Could you check a few things on this model? Use its own coordinates, in mm. Face numbers are marked on the shaded views. Coordinates: 2 decimals unless noted, no trailing zeros. Order: outer loops, then holes, each group sorted by start corner. A loop starts at its lowest first (then second) coordinate and runs counter-clockwise, first axis right, second up. Notation, with made-up numbers: (74.5, 69.5) -> (97.5, 69.5) arc R27 ccw to (97.5, 104.5) -> close; hole circle Ø4 at (-21.5, 67.25). An arc over 180 degrees is marked (long way). Put each result on its own line as item: value. Start each with the question number.
Q1. If we section it at D-D (z = -10.5): Please give me the cut outline in (x, y), and give its area (3 significant figures).
Q2. Please list where these lines run through material, in increasing order: line 1 along Z through (x, y) = (-6, 6.4); line 2 along X through (y, z) = (5.6, -10.5); line 3 along Z through (x, y) = (-10.5, 3.5).
Q3. We'd pull the mould along Z, two halves only. Please class the marked faces 1, 2 and 3: +Z half, -Z half, draft (parallel to the pull), parting line (faces both ways), or undercut.
Q4. If we section it at B-B (y = 3.25): Please give me the cut outline in (x, z), and give its area (3 significant figures).
Q5. If we section it at C-C (x = -12): Please give me the cut outline in (y, z), and give its area (3 significant figures).
Q6. If we section it at A-A (y = 8.5): Please give me the cut outline in (x, z).
Q7. Will these pins go through, and if not, where does the flat tip stop? pin 1 (2 mm diameter, centred on y = 1.5, z = -6.5, fed in from -X); pin 2 (0.9 mm diameter, centred on x = 5.5, z = -10, fed in from +Y).
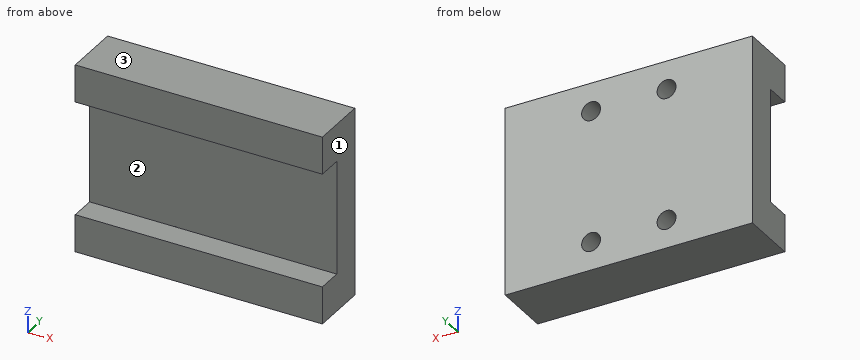
from build123d import *

# Parameters (mm, degrees)
SKETCH_1_W          = 39.3
SKETCH_1_H          = 30
EXTRUDE_1_DEPTH     = 9
SKETCH_2_W          = 39.3
SKETCH_2_H          = 18.1
CUT_EXTRUDE_1_DEPTH = 4
SKETCH_3_R          = 1.5
CUT_EXTRUDE_2_DEPTH = 5


with BuildPart() as part:
    # 草图1 → 凸台-拉伸1 (new body)
    with BuildSketch(Plane(origin=(0, 0, 0), x_dir=(1, 0, 0), z_dir=(0, 1, 0))):
        Rectangle(SKETCH_1_W, SKETCH_1_H)
    extrude(amount=EXTRUDE_1_DEPTH)

    # 草图2 → 切除-拉伸1 (cut)
    with BuildSketch(Plane.XZ):
        Rectangle(SKETCH_2_W, SKETCH_2_H)
    extrude(amount=-CUT_EXTRUDE_1_DEPTH, mode=Mode.SUBTRACT)

    # 草图3 → 切除-拉伸2 (cut)
    with BuildSketch(Plane(origin=(0, 9, 0), x_dir=(1, 0, 0), z_dir=(0, 1, 0))):
        with Locations((-6, 10.5)):
            Circle(SKETCH_3_R)
        with Locations((6, 10.5)):
            Circle(SKETCH_3_R)
        with Locations((6, -10.5)):
            Circle(SKETCH_3_R)
        with Locations((-6, -10.5)):
            Circle(SKETCH_3_R)
    extrude(amount=-CUT_EXTRUDE_2_DEPTH, mode=Mode.SUBTRACT)


solid = part.part
The answers:
1. outline: (-19.65, 0) -> (19.65, 0) -> (19.65, 9) -> (7.5, 9) -> (7.5, 4) -> (4.5, 4) -> (4.5, 9) -> (-4.5, 9) -> (-4.5, 4) -> (-7.5, 4) -> (-7.5, 9) -> (-19.65, 9) -> close
1. area: 324 mm^2
2. line 1: -15 to -12, -9 to 9, 12 to 15
2. line 2: -19.65 to -7.5, -4.5 to 4.5, 7.5 to 19.65
2. line 3: -15 to -9.05, 9.05 to 15
3. face 1: draft
3. face 2: undercut
3. face 3: +Z half
4. outline: (-19.65, -15) -> (19.65, -15) -> (19.65, -9.05) -> (-19.65, -9.05) -> close; (-19.65, 9.05) -> (19.65, 9.05) -> (19.65, 15) -> (-19.65, 15) -> close
4. area: 468 mm^2
5. outline: (0, -15) -> (9, -15) -> (9, 15) -> (0, 15) -> (0, 9.05) -> (4, 9.05) -> (4, -9.05) -> (0, -9.05) -> close
5. area: 198 mm^2
6. outline: (-19.65, -15) -> (19.65, -15) -> (19.65, 15) -> (-19.65, 15) -> close; hole circle Ø3 at (-6, -10.5); hole circle Ø3 at (-6, 10.5); hole circle Ø3 at (6, -10.5); hole circle Ø3 at (6, 10.5)
7. pin 1: through
7. pin 2: y = 4
